Here's how the part is built. I have some questions about the finished solid (model axes, mm). Give positions to 0.01 mm unless a question says otherwise; leave off trailing zeros. Write each loop counter-clockwise with the first axis right and the second up, starting at its lowest first coordinate (ties: lowest second). Pieces come first, ordered by that corner, then holes. Notation, with made-up numbers: (59.5, 36.5) -> (113.5, 36.5) arc R27 ccw to (113.5, 66.5) -> close; hole circle Ø10 at (-12.5, -15.5). An arc over 180 degrees is marked (long way). Use CSV: the item, a comma, the result in double quotes. Start each with the question number.
(1) If we mould it in two halves opening along Y, with no side actions, what happens to faces 1 (the cylindrical face through (112.444, 10.691, 19.727)), 2 (the flat face through (59, 0, 19)), 3 (the flat face through (59, 10, 0)), 4 (the cylindrical face through (8.1, 11.6, 19.7))? For each: pulls with the +Y half, pulls with the -Y half, needs draft (parallel to the pull), parting line crosses it, or undercut.
(2) I need wall thicknesses on L1, parallel to X at y = 10, z = 25; L2, parallel to X at y = 11, z = 26; L3, parallel to Y at x = 9.75, z = 12. Which ranges of each line are inside material? Lowest first, please. Write a range as [from, to].
(3) Suppose I cut it at B-B on z = 8. List the corners of the cut face in (x, y) for me.
(4) Suppose I cut it at C-C on y = 10. List the corners of the cut face in (x, z) for me, plus the area to 3 significant figures.
(5) Suppose I cut it at A-A on x = 110.25. List the corners of the cut face in (y, z) for me.
(6) For pin 1 Ø5 at (y, z) = (2, 31) entering from +X; pin 2 Ø3.5 at (x, y) = (110.25, 10) entering from -Z; pin 3 Ø3 at (y, z) = (2, 15.5) entering from +X, each with a flat end and sliding along its axis, tell me the tip position at first contact or that it passes through.
from build123d import *

# Parameters (mm, degrees)
CYLINDER_R        = 2.3
CYLINDER_DEPTH    = 50
CYLINDER001_R     = 2.3
CYLINDER001_DEPTH = 50
BOX_W             = 120
BOX_H             = 20
BOX_DEPTH         = 39.5
FILLET_R          = 5
CHAMFER_SIZE      = 0.5


with BuildPart() as cylinder:
    # Cylinder → Cylinder (new body)
    with BuildSketch(Plane(origin=(9.75, 10, -1), x_dir=(1, 0, 0), z_dir=(0, 0, 1))):
        Circle(CYLINDER_R)
    extrude(amount=CYLINDER_DEPTH)


with BuildPart() as fusion:
    # Cylinder001 → Cylinder001 (new body)
    with BuildSketch(Plane(origin=(110.25, 10, -1), x_dir=(1, 0, 0), z_dir=(0, 0, 1))):
        Circle(CYLINDER001_R)
    extrude(amount=CYLINDER001_DEPTH)

    # Fusion: union Cylinder
    add(cylinder.part)


with BuildPart() as chamfer_body:
    # Box → Box (new body)
    with BuildSketch(Plane.XY):
        with Locations((60, 10)):
            Rectangle(BOX_W, BOX_H)
    extrude(amount=BOX_DEPTH)

    # Cut: cut Fusion
    add(fusion.part, mode=Mode.SUBTRACT)

    # Fillet
    fillet_edges = [chamfer_body.edges().sort_by_distance(p)[0] for p in [
        (0, 0, 19.75),
        (0, 20, 19.75),
        (120, 0, 19.75),
        (120, 20, 19.75),
    ]]
    fillet(fillet_edges, radius=FILLET_R)

    # Chamfer
    chamfer_edges = [chamfer_body.edges().sort_by_distance(p)[0] for p in [
        (107.95, 10, 0),
        (7.45, 10, 0),
    ]]
    chamfer(chamfer_edges, length=CHAMFER_SIZE)


solid = chamfer_body.part
Geometry says:
1,face 1,"undercut"
1,face 2,"pulls with the -Y half"
1,face 3,"needs draft"
1,face 4,"undercut"
2,L1,"[0, 7.45], [12.05, 107.95], [112.55, 120]"
2,L2,"[0, 7.68], [11.82, 108.18], [112.32, 120]"
2,L3,"[0, 7.7], [12.3, 20]"
3,outline,"(0, 5) arc R5 ccw to (5, 0) -> (115, 0) arc R5 ccw to (120, 5) -> (120, 15) arc R5 ccw to (115, 20) -> (5, 20) arc R5 ccw to (0, 15) -> close; hole circle Ø4.6 at (9.75, 10); hole circle Ø4.6 at (110.25, 10)"
4,outline,"(0, 0) -> (6.95, 0) -> (7.45, 0.5) -> (7.45, 39.5) -> (0, 39.5) -> close; (12.05, 0.5) -> (12.55, 0) -> (107.45, 0) -> (107.95, 0.5) -> (107.95, 39.5) -> (12.05, 39.5) -> close; (112.55, 0.5) -> (113.05, 0) -> (120, 0) -> (120, 39.5) -> (112.55, 39.5) -> close"
4,area,"4,380 mm²"
5,outline,"(0, 0) -> (7.2, 0) -> (7.7, 0.5) -> (7.7, 39.5) -> (0, 39.5) -> close; (12.3, 0.5) -> (12.8, 0) -> (20, 0) -> (20, 39.5) -> (12.3, 39.5) -> close"
6,pin 1,"x = 119.97"
6,pin 2,"through"
6,pin 3,"x = 119.77"
